The model under review builds one solid part; all positions refer to its coordinate system, in mm. A direction names the side the tool comes from. Round coordinates to 2 decimals unless told otherwise and drop trailing zeros. Write each loop counter-clockwise with the first axis right and the second up, starting at its lowest first coordinate (ties: lowest second). Pieces come first, ordered by that corner, then holes. Notation, with made-up numbers: M -26,-14.5 L -5,-14.5 A25 cw -5,-1.5 Z; hole C 82.5,-39.75 d6. An arc over 180 degrees is marked long. Write item = value, one per line. Start each with the question number.
Item 1: Take a section at A-A, the plane x = -8. Give the boundary of the cut face in (y, z), plus the area to 3 significant figures.
Item 2: Tool access review of faces 3 (the cylindrical face through (-42.51, 1.01, 14.21)), 4 (the flat face through (-1, 2, -3)): name each direction out of +Z, -Z, +X, -X, +Y, -Y from which nothing blocks a thin tool from reaching the whole face with its end or side.
Item 3: To check wall thickness, follow line 1 along X through (y, z) = (1.4, -16); line 2 along Z through (x, y) = (44.5, 1.3); line 3 along X through (y, z) = (0.5, 6.5). State the ranges of each line that lie inside material, in increasing order.
Item 4: For pin 1 Ø1 at (y, z) = (0.5, 23.5) entering from -X; pin 2 Ø1 at (x, y) = (-1.5, 1.5) entering from -Z; pin 3 Ø0.6 at (y, z) = (1, 23) entering from +X, all flat-tipped, find the tip position at first contact; note any pin that passes through.
Item 5: Take a section at B-B, the plane y = 1.5. Give the number of separate pieces and of enclosed holes in the cut face, plus the area to 3 significant figures.
Item 6: The part is to be moulded in two halves that separate along X. For faces 1 (the flat face through (-1, 0, -3)), 2 (the cylindrical face through (-67.38, 1.01, 11.7)), say which applies: +X half, -X half, draft (parallel to the pull), parting line (faces both ways), or undercut.
from build123d import *

# Parameters (mm, degrees)
SKETCH_1_W          = 147
SKETCH_1_H          = 40
EXTRUDE_1_DEPTH     = 2
CUT_EXTRUDE_1_DEPTH = 77.198753271
SKETCH_3_R          = 1
CUT_EXTRUDE_2_DEPTH = 77.198753271
SKETCH_5_W          = 12
SKETCH_5_H          = 2
EXTRUDE_2_DEPTH     = 5
SKETCH_7_R          = 1
CUT_EXTRUDE_3_DEPTH = 78.661122835
CUT_EXTRUDE_5_DEPTH = 78.661122835
SKETCH_11_W         = 26
SKETCH_11_H         = 3.5
CUT_EXTRUDE_6_DEPTH = 10
FILLET_1_R          = 2
CUT_EXTRUDE_7_DEPTH = 78.661122835


with BuildPart() as part:
    # 草图1 → 凸台-拉伸1 (new body)
    with BuildSketch(Plane(origin=(0, 0, 0), x_dir=(1, 0, 0), z_dir=(0, 1, 0))):
        Rectangle(SKETCH_1_W, SKETCH_1_H)
    extrude(amount=EXTRUDE_1_DEPTH)

    # 草图2 → 切除-拉伸1 (cut, through all)
    with BuildSketch(Plane(origin=(0, 2, 0), x_dir=(1, 0, 0), z_dir=(0, 1, 0))):
        Polygon((-45.658720859, -7.223049229), (-45.42875824, -5.035101059), (-30.51092981, -6.603028008), (-30.740892429, -8.790976178), align=None)
    cut_extrude_1 = extrude(amount=-CUT_EXTRUDE_1_DEPTH, mode=Mode.SUBTRACT)

    # 草图3 → 切除-拉伸2 (cut, through all)
    with BuildSketch(Plane(origin=(0, 2, 0), x_dir=(1, 0, 0), z_dir=(0, 1, 0))):
        with Locations((-44.434236345, -5.139629522)):
            Circle(SKETCH_3_R)
        with Locations((-44.664198964, -7.327577692)):
            Circle(SKETCH_3_R)
        with Locations((-31.505451705, -6.498499545)):
            Circle(SKETCH_3_R)
        with Locations((-31.735414324, -8.686447714)):
            Circle(SKETCH_3_R)
    cut_extrude_2 = extrude(amount=-CUT_EXTRUDE_2_DEPTH, mode=Mode.SUBTRACT)

    # 镜向1: 切除-拉伸1, 切除-拉伸2 across plane
    add(cut_extrude_1.mirror(Plane(origin=(0, 0, 0), x_dir=(0, 0, 1), z_dir=(1, 0, 0))), mode=Mode.SUBTRACT)
    add(cut_extrude_2.mirror(Plane(origin=(0, 0, 0), x_dir=(0, 0, 1), z_dir=(1, 0, 0))), mode=Mode.SUBTRACT)

    # 草图5 → 凸台-拉伸2 (add)
    with BuildSketch(Plane.XY.offset(20)):
        with Locations((53.5, 1)):
            Rectangle(SKETCH_5_W, SKETCH_5_H)
        with Locations((-53.5, 1)):
            Rectangle(SKETCH_5_W, SKETCH_5_H)
    extrude(amount=EXTRUDE_2_DEPTH)

    # 草图7 → 切除-拉伸3 (cut, through all)
    with BuildSketch(Plane(origin=(0, 2, 0), x_dir=(1, 0, 0), z_dir=(0, 1, 0))):
        with Locations((60.5, -20)):
            Circle(SKETCH_7_R)
        with Locations((46.5, -20)):
            Circle(SKETCH_7_R)
        with Locations((-46.5, -20)):
            Circle(SKETCH_7_R)
        with Locations((-60.5, -20)):
            Circle(SKETCH_7_R)
    extrude(amount=-CUT_EXTRUDE_3_DEPTH, mode=Mode.SUBTRACT)

    # 草图10 → 切除-拉伸5 (cut, through all)
    with BuildSketch(Plane(origin=(0, 2, 0), x_dir=(1, 0, 0), z_dir=(0, 1, 0))):
        with BuildLine():
            Line((-64.629116749, -9.423125996), (-44.738678842, -11.513695262))
            ThreePointArc((-44.738678842, -11.513695262), (-42.513695262, -14.261321158), (-45.261321158, -16.486304738))
            Line((-45.261321158, -16.486304738), (-65.151759066, -14.395735473))
            ThreePointArc((-65.151759066, -14.395735473), (-67.376742646, -11.648109576), (-64.629116749, -9.423125996))
        make_face()
    cut_extrude_5 = extrude(amount=-CUT_EXTRUDE_5_DEPTH, mode=Mode.SUBTRACT)

    # 镜向2: 切除-拉伸5 across plane
    add(cut_extrude_5.mirror(Plane(origin=(0, 0, 0), x_dir=(0, 0, 1), z_dir=(1, 0, 0))), mode=Mode.SUBTRACT)

    # 草图11 → 切除-拉伸6 (cut)
    with BuildSketch(Plane(origin=(0, 2, 0), x_dir=(1, 0, 0), z_dir=(0, 1, 0))):
        with Locations((0, 20)):
            Rectangle(SKETCH_11_W, SKETCH_11_H)
    extrude(amount=-CUT_EXTRUDE_6_DEPTH, mode=Mode.SUBTRACT)

    # 圆角1
    # the kernel refuses this fillet: 2 mm, written as the material it takes off along each edge
    with BuildSketch(Plane(origin=(13, -4.960783708, -20), x_dir=(1, 0, 0), z_dir=(0, 1, 0)), Plane(origin=(-13, 6.960783708, -20), x_dir=(-1, 0, 0), z_dir=(0, -1, 0))) as fillet_1_piece_1:
        with BuildLine():
            CenterArc((1.984313483, -2), FILLET_1_R, 90, 82.819244219)
            Line((0, -1.75), (-0.03968627, -1.745))
            ThreePointArc((-0.03968627, -1.745), (-0.04, -0.875), (-0.04, 0))
            Line((-0.04, 0), (0, 0.04))
            Line((0, 0.04), (1.984313483, 0.04))
            Line((1.984313483, 0.04), (1.984313483, 0))
        make_face()
    extrude(amount=11.921567416, mode=Mode.SUBTRACT)

    # 草图12 → 切除-拉伸7 (cut, through all)
    with BuildSketch(Plane(origin=(0, 2, 0), x_dir=(1, 0, 0), z_dir=(0, 1, 0))):
        with BuildLine():
            Line((-6.25, 16), (-6.25, 13))
            ThreePointArc((-6.25, 13), (-8, 11.25), (-9.75, 13))
            Line((-9.75, 13), (-9.75, 16))
            ThreePointArc((-9.75, 16), (-8, 17.75), (-6.25, 16))
        make_face()
        with BuildLine():
            Line((9.75, 16), (9.75, 13))
            ThreePointArc((9.75, 13), (8, 11.25), (6.25, 13))
            Line((6.25, 13), (6.25, 16))
            ThreePointArc((6.25, 16), (8, 17.75), (9.75, 16))
        make_face()
    extrude(amount=-CUT_EXTRUDE_7_DEPTH, mode=Mode.SUBTRACT)


solid = part.part
Response values:
q1.outline = M 0,-18.25 L 2,-18.25 L 2,-17.75 L 0,-17.75 Z; M 0,-11.25 L 2,-11.25 L 2,20 L 0,20 Z
q1.area = 63.5 mm2
q2.face_3 = +Y, -Y
q2.face_4 = +Z, -Z, +X, -X, +Y
q3.line_1 = -73.5 to -9.75, -6.25 to 6.25, 9.75 to 73.5
q3.line_2 = -20 to 4.14, 8.31 to 11.55, 16.45 to 20
q3.line_3 = -73.5 to -45.58, -30.51 to 30.51, 45.58 to 73.5
q4.pin_1 = -59.5
q4.pin_2 = -18.25
q4.pin_3 = 59.5
q5.separate_pieces = 1
q5.enclosed_holes = 6
q5.area = 5,590 mm2
q6.face_1 = draft
q6.face_2 = undercut
